Answer from the drawing. Dimensions are ordinates in mm from the lowest x, y and z of the part. Round coordinates to 2 decimals unless told otherwise and drop trailing zeros. Write each loop counter-clockwise with the first axis right and the second up, starting at its lowest first coordinate (ties: lowest second). Pieces come first, ordered by that corner, then holes. Notation, with made-up numbers: (41, 34) -> (68, 34) arc R32 ccw to (68, 72) -> close; hole circle Ø2 at (22, 34.25). An arc over 180 degrees is marked (long way). Return JSON: item names as keys, results as strings. Group by question number.
(1) Given pin 1 (2 mm diameter, centred on x = 1.5, z = 1.5, fed in from -Y); pin 2 (2 mm diameter, centred on x = 2.5, z = 2, fed in from +Y), each flat-ended and moving along its own axis, determine where each tip first touches the part or whether it passes through.
(2) A straight line is drawn through the part: line 1 (X direction, y = 41, z = 0.4). Find the intervals that lie inside material, in ascending order.
(3) A cutting plane is placed at A-A on z = 1.9. Give the vertices of the cut face in (x, y).
(4) A cutting plane is placed at B-B on y = 126. Give the vertices of the cut face in (x, z).
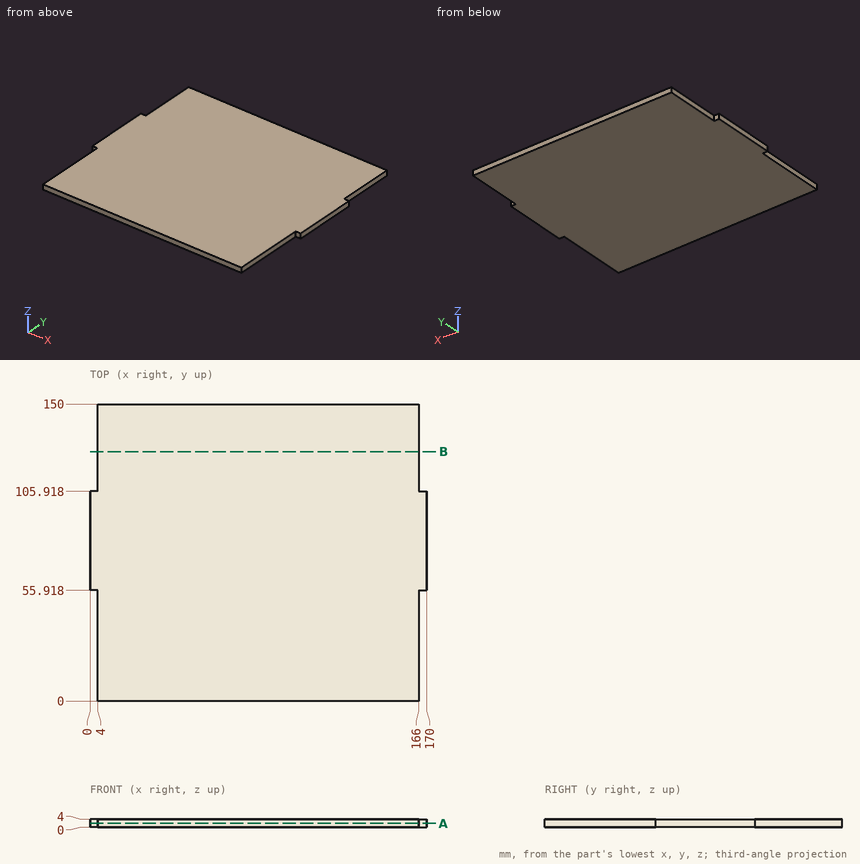
Checks:
{
 "1": {"pin 1": "stops at y = 55.92", "pin 2": "stops at y = 105.92"},
 "2": {"line 1": "x = 4 to 166"},
 "3": {"outline": "(0, 55.92) -> (4, 55.92) -> (4, 0) -> (166, 0) -> (166, 55.92) -> (170, 55.92) -> (170, 105.92) -> (166, 105.92) -> (166, 150) -> (4, 150) -> (4, 105.92) -> (0, 105.92) -> close"},
 "4": {"outline": "(4, 0) -> (166, 0) -> (166, 4) -> (4, 4) -> close"}
}
